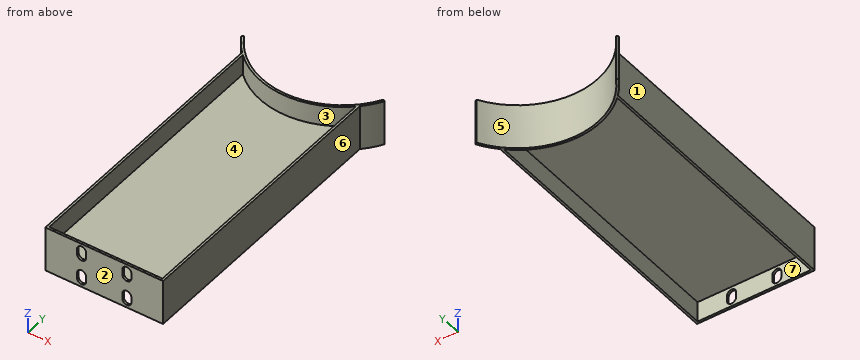
Autodesk Inventor part; units mm, degrees
ref_plane "YZ Plane" through (0, 0, 0) normal (1, 0, 0) x (0, 1, 0)
ref_plane "XZ Plane" through (0, 0, 0) normal (0, 1, 0) x (-1, 0, 0)
ref_plane "XY Plane" through (0, 0, 0) normal (0, 0, 1) x (1, 0, 0)
sketch "Sketch1" plane through (0, 0, 0) normal (0, 0, 1) x (1, 0, 0)
  line L0 (-130, 607) -> (-130, 0)
  line L1 (-130, 0) -> (130, 0)
  line L2 (130, 0) -> (130, 607)
  line L3 (125, 5) -> (125, 602.1317)
  line L4 (-125, 5) -> (-125, 602.1317)
  line L5 (-125, 5) -> (125, 5)
  arc A0 (-153.9793, 646.614) -> (153.9793, 646.614) centre (0, 735.514) ccw
  arc A1 (130, 607) -> (158.3094, 644.114) centre (0, 735.514) ccw
  arc A2 (-158.3094, 644.114) -> (-130, 607) centre (0, 735.514) ccw
  arc A3 (-125, 602.1317) -> (125, 602.1317) centre (0, 735.514) ccw
  line L6 (-158.3094, 644.114) -> (-153.9793, 646.614)
  line L7 (153.9793, 646.614) -> (158.3094, 644.114)
  point P0 (0, 0)
  point P1 (0, 0)
  point P2 (0, 5)
  dimension "d0" = 260
  dimension "d2" = 607
  dimension "d3" = 607
  dimension "d6" = 5
  dimension "d7" = 5
  dimension "d8" = 5
  dimension "d57" = 355.6
  dimension "d61" = 5
  dimension "d64" = 182.8
  dimension "d79" = 130
  dimension "d80" = 120
  dimension "d81" = 158.3094
  dimension "d82" = 153.9793
  dimension "d83" = 153.9793
extrude "Extrusion1" add sketch "Sketch1" along normal mid plane 100
sketch "Sketch5" plane through (0, 0, 0) normal (0, 0, 1) x (1, 0, 0)
  line L0 (-125, 602.1317) -> (-125, 5)
  line L1 (-125, 602.1317) -> (-125, 5)
  line L2 (-125, 5) -> (125, 5)
  line L3 (-125, 5) -> (125, 5)
  line L4 (125, 5) -> (125, 602.1317)
  line L5 (125, 5) -> (125, 602.1317)
  arc A0 (-125, 602.1317) -> (125, 602.1317) centre (0, 735.514) ccw
  point P0 (0, 0)
  point P1 (0, 5)
  dimension "d67" = 365.6
extrude "Extrusion2" add sketch "Sketch5" along normal mid plane 10
sketch "Sketch6" plane through (-130, 0, 50) normal (0, -1, 0) x (1, 0, 0)
  line L0 (5, -100) -> (255, -100)
  line L1 (130, -100) -> (130, 0)
  line L2 (0, 0) -> (260, 0)
  line L3 (80, -16) -> (80, -28.5) construction
  line L4 (70, -16) -> (70, -28.5)
  line L5 (90, -28.5) -> (90, -16)
  arc A0 (90, -16) -> (70, -16) centre (80, -16) ccw
  arc A1 (70, -28.5) -> (90, -28.5) centre (80, -28.5) ccw
  line L6 (80, -71.5) -> (80, -84) construction
  line L7 (70, -71.5) -> (70, -84)
  line L8 (90, -84) -> (90, -71.5)
  arc A2 (90, -71.5) -> (70, -71.5) centre (80, -71.5) ccw
  arc A3 (70, -84) -> (90, -84) centre (80, -84) ccw
  line L9 (180, -16) -> (180, -28.5) construction
  line L10 (190, -16) -> (190, -28.5)
  line L11 (170, -28.5) -> (170, -16)
  arc A4 (190, -16) -> (170, -16) centre (180, -16) ccw
  arc A5 (170, -28.5) -> (190, -28.5) centre (180, -28.5) ccw
  line L12 (180, -71.5) -> (180, -84) construction
  line L13 (190, -71.5) -> (190, -84)
  line L14 (170, -84) -> (170, -71.5)
  arc A6 (190, -71.5) -> (170, -71.5) centre (180, -71.5) ccw
  arc A7 (170, -84) -> (190, -84) centre (180, -84) ccw
  point P0 (130, -50)
  point P1 (80, -22.25)
  point P2 (80, -77.75)
  point P3 (180, -22.25)
  point P4 (180, -77.75)
  dimension "d88" = 100
  dimension "d89" = 10
  dimension "d90" = 100
  dimension "d92" = 10
  dimension "d93" = 68
  dimension "d94" = 16
  dimension "d95" = 43
  dimension "d96" = 12.5
extrude "Extrusion5" cut sketch "Sketch6" against normal blind 10
properties part number "Fix Saddle new 1" material "Steel ASTM A36"
Source: CAD feature listing. Evaluate the final solid. Frame: model axes, mm. Face numbers are marked on the shaded views. A direction names the side the tool comes from. Round coordinates to 2 decimals unless told otherwise and drop trailing zeros. Loops run counter-clockwise (first coordinate to the right, second up) from the corner with the lowest first, then second, coordinate; pieces in that order, holes last. Notation, with made-up numbers: (59.25, 87) - (110.25, 87) arc R19 cw to (110.25, 120) - close; hole circle Ø2 at (28.25, -21). An arc over 180 degrees is marked (long way). Use CSV: the item, a comma, the result in double quotes.
Q1. Reachability of the marked faces 4, 5, 6 and 7 from +Z, -Z, +X, -X, +Y, -Y: full face, straight path, thin tool, end or side. Return the list, or none.
Reported:
face 4,"+Z"
face 5,"+Z, -Z, +Y"
face 6,"+Z, -Z, +X, -Y"
face 7,"-Z"
Q2. Section query A-A, the plane x = -50. Output: boundary loops of the cut face in (y, z) (3 decimals), then the cut area to 3 significant figures.
Reported:
outline,"(0, -50) - (5, -50) - (5, -44) - (0, -44) - close; (0, -11.5) - (5, -11.5) - (5, -5) - (559.685, -5) - (559.685, -50) - (564.889, -50) - (564.889, 50) - (559.685, 50) - (559.685, 5) - (5, 5) - (5, 11.5) - (0, 11.5) - close; (0, 44) - (5, 44) - (5, 50) - (0, 50) - close"
area,"6,240 mm^2"
Q3. Pin query (flat end, axial travel): pin 1 Ø3 at (x, z) = (50.5, 12.5) entering from +Y; pin 2 Ø13.5 at (y, z) = (403, 32) entering from +X; pin 3 Ø2 at (y, z) = (299.5, -33.5) entering from -X. Return the tip coordinate at first contact, or that it passes through.
Reported:
pin 1,"y = 565.49"
pin 2,"x = 130"
pin 3,"x = -130"
Q4. Section query B-B, the plane y = 452. Output: boundary loops of the cut face in (x, z), then the cut area to 3 significant figures.
Reported:
outline,"(-130, -50) - (-125, -50) - (-125, -5) - (125, -5) - (125, -50) - (130, -50) - (130, 50) - (125, 50) - (125, 5) - (-125, 5) - (-125, 50) - (-130, 50) - close"
area,"3,500 mm^2"
Q5. Section query C-C, the plane x = 66. Output: boundary loops of the cut face in (y, z).
Reported:
outline,"(0, -50) - (5, -50) - (5, -5) - (565.04, -5) - (565.04, -50) - (570.42, -50) - (570.42, 50) - (565.04, 50) - (565.04, 5) - (5, 5) - (5, 50) - (0, 50) - close"
Q6. Mould query, pull axis X, two halves, no side actions, for the marked faces 1, 2 and 3. Classes: pulls with the +X half, pulls with the -X half, needs draft (parallel to the pull), parting line crosses it, or undercut.
Reported:
face 1,"pulls with the -X half"
face 2,"needs draft"
face 3,"undercut"
Q7. Ray query, line 1 along X through (y, z) = (163.5, -31); line 2 along X through (y, z) = (387.5, -2); line 3 along Z through (x, y) = (113, 48.5). Return the intervals inside material, ascending.
Reported:
line 1,"-130 to -125, 125 to 130"
line 2,"-130 to 130"
line 3,"-5 to 5"
